```python
from build123d import *

# Parameters (mm, degrees)
SALIENTE_EXTRUIR1_DEPTH = 160
CHAFL_N1_SIZE           = 1.5
CROQUIS2_R              = 2.25
CORTAR_EXTRUIR1_DEPTH   = 320


with BuildPart() as part:
    # Croquis1 → Saliente-Extruir1 (new body, symmetric)
    with BuildSketch(Plane(origin=(0, 0, 0), x_dir=(0, 0, -1), z_dir=(1, 0, 0))):
        Polygon((-15, 0), (15, 0), (15, 5), (20, 5), (20, -5), (-20, -5), (-20, 5), (-15, 5), align=None)
    extrude(amount=SALIENTE_EXTRUIR1_DEPTH, both=True)

    # Chaflán1
    chafl_n1_edges = [part.edges().sort_by_distance(p)[0] for p in [
        (0, 5, -20),
        (0, -5, -20),
        (0, -5, 20),
        (0, 5, 20),
        (0, 5, 15),
    ]]
    chamfer(chafl_n1_edges, length=CHAFL_N1_SIZE)

    # Croquis2 → Cortar-Extruir1 (cut)
    with BuildSketch(Plane(origin=(0, 0, 0), x_dir=(1, 0, 0), z_dir=(0, 1, 0))):
        with Locations((-146, 0)):
            Circle(CROQUIS2_R)
        with Locations((-131, 0)):
            Circle(CROQUIS2_R)
        with Locations((131, 0)):
            Circle(CROQUIS2_R)
        with Locations((146, 0)):
            Circle(CROQUIS2_R)
    extrude(amount=-CORTAR_EXTRUIR1_DEPTH, mode=Mode.SUBTRACT)


solid = part.part
```
Geometry check sheet. Reference: the model listing, model coordinates, mm. A direction names the side the tool comes from. Give positions to 0.01 mm unless a question says otherwise; leave off trailing zeros. Order: outer loops, then holes, each group sorted by start corner. A loop starts at its lowest first (then second) coordinate and runs counter-clockwise, first axis right, second up. Notation, with made-up numbers: (31, 34) - (35, 34) arc R14 cw to (35, 43) - close; hole circle Ø2 at (-25, 69.5). An arc over 180 degrees is marked (long way). Write item = value, one per line. Start each with the question number.
1) Draft check along Z on faces 1 (the flat face through (2, 0, -20)), 2 (the flat face through (-160, -2, 0)), 3 (the flat face through (2, 2, -15)). Enter one of: released by +Z, released by -Z, zero draft, split by the parting line, or undercut.
2) Gauge pin test, flat end, axial feed: pin 1 Ø7 at (x, z) = (-146, 0) entering from -Y. Record the tip position at first contact, or that the pin passes through.
3) Scan lines: L1, parallel to X at y = -3.6, z = 0; L2, parallel to Z at x = 131, y = -2.35; L3, parallel to Z at x = -12, y = 2.25. Record each from-to range of solid material in increasing order.
4) Access from +Z, -Z, +X, -X, +Y, -Y to the whole of each face (thin tool, end or side, straight path). Record for faces 4 (the flat face through (2, 0, 0)), 5 (the flat face through (2, -5, 0)).
5) Section check A-A (x = -24). Enter the section's corners in (y, z).
6) Section check B-B (z = 6.5). Enter the section's corners in (x, y).
Geometry check:
q1.face_1 = released by -Z
q1.face_2 = zero draft
q1.face_3 = undercut
q2.pin_1 = -5
q3.L1 = -160 to -148.25, -143.75 to -133.25, -128.75 to 128.75, 133.25 to 143.75, 148.25 to 160
q3.L2 = -20 to -2.25, 2.25 to 20
q3.L3 = -20 to -15, 15 to 20
q4.face_4 = +X, -X, +Y
q4.face_5 = +Z, -Z, +X, -X, -Y
q5.outline = (-5, -18.5) - (-3.5, -20) - (3.5, -20) - (5, -18.5) - (5, -15) - (0, -15) - (0, 15) - (3.5, 15) - (5, 16.5) - (5, 18.5) - (3.5, 20) - (-3.5, 20) - (-5, 18.5) - close
q6.outline = (-160, -5) - (160, -5) - (160, 0) - (-160, 0) - close
